Here's how the part is built. I have some questions about the finished solid (model axes, mm). Give positions to 0.01 mm unless a question says otherwise; leave off trailing zeros. Loops run counter-clockwise (first coordinate to the right, second up) from the corner with the lowest first, then second, coordinate; pieces in that order, holes last. Notation, with made-up numbers: (-27.5, -22.75) -> (-10.5, -22.75) arc R34 cw to (-10.5, 14.25) -> close; hole circle Ø5 at (54.5, -9). An arc over 180 degrees is marked (long way). Answer in a Markdown table with one row per item. Add a question column.
Item 1: We'd pull the mould along X, two halves only. Please class faces 1 (the face through (7.5, 1, 0)), 2 (the face through (-7.5, 1, 0)), 3 (the face through (-4.928, 0.811, -0.18)): released by +X, released by -X, zero draft, split by the parting line, or undercut.
Item 2: If we section it at A-A (z = 0): Write out the boundary of the cut face in (x, y).
Item 3: If we section it at B-B (x = -5.5): Write out the boundary of the cut face in (y, z), then the cut area to 3 significant figures.
Item 4: If I drill on line 1 (X direction, y = 0.9, z = 0); line 2 (Z direction, x = -5.5, y = 0.35); line 3 (Z direction, x = -5.25, y = 0.3), over which ranges is the centre line in solid material (lowest first)?
Item 5: If we section it at C-C (y = 0.4): Write out the boundary of the cut face in (x, z).
```python
from build123d import *

# Parameters (mm, degrees)
SKETCH1_W           = 15
SKETCH1_H           = 4
BOSS_EXTRUDE1_DEPTH = 1.6
SKETCH5_W           = 15
SKETCH5_H           = 1.6
BOSS_EXTRUDE4_DEPTH = 1.5
SKETCH6_W           = 15
SKETCH6_H           = 1.6
BOSS_EXTRUDE5_DEPTH = 0.9
SKETCH8_R           = 0.6
CUT_EXTRUDE1_DEPTH  = 10


with BuildPart() as part:
    # Sketch1 → Boss-Extrude1 (new body)
    with BuildSketch(Plane(origin=(0, 0, 0), x_dir=(1, 0, 0), z_dir=(0, 1, 0))):
        Rectangle(SKETCH1_W, SKETCH1_H)
    extrude(amount=BOSS_EXTRUDE1_DEPTH)

    # Sketch5 → Boss-Extrude4 (add)
    with BuildSketch(Plane.XY.offset(2)):
        with Locations((0, 0.8)):
            Rectangle(SKETCH5_W, SKETCH5_H)
    extrude(amount=BOSS_EXTRUDE4_DEPTH)

    # Sketch6 → Boss-Extrude5 (add)
    with BuildSketch(Plane(origin=(0, 0, -2), x_dir=(-1, 0, 0), z_dir=(0, 0, -1))):
        with Locations((0, 0.8)):
            Rectangle(SKETCH6_W, SKETCH6_H)
    extrude(amount=BOSS_EXTRUDE5_DEPTH)

    # Sketch8 → Cut-Extrude1 (cut)
    with BuildSketch(Plane(origin=(0, 1.6, 0), x_dir=(1, 0, 0), z_dir=(0, 1, 0))):
        with Locations((5.5, 0)):
            Circle(SKETCH8_R)
        with Locations((-5.5, 0)):
            Circle(SKETCH8_R)
    extrude(amount=-CUT_EXTRUDE1_DEPTH, mode=Mode.SUBTRACT)


solid = part.part
```
Recorded:
| question | item | result |
|---|---|---|
| 1 | face 1 | released by +X |
| 1 | face 2 | released by -X |
| 1 | face 3 | undercut |
| 2 | outline | (-7.5, 0) -> (-6.1, 0) -> (-6.1, 1.6) -> (-7.5, 1.6) -> close; (-4.9, 0) -> (4.9, 0) -> (4.9, 1.6) -> (-4.9, 1.6) -> close; (6.1, 0) -> (7.5, 0) -> (7.5, 1.6) -> (6.1, 1.6) -> close |
| 3 | outline | (0, -2.9) -> (1.6, -2.9) -> (1.6, -0.6) -> (0, -0.6) -> close; (0, 0.6) -> (1.6, 0.6) -> (1.6, 3.5) -> (0, 3.5) -> close |
| 3 | area | 8.32 mm^2 |
| 4 | line 1 | x = -7.5 to -6.1, -4.9 to 4.9, 6.1 to 7.5 |
| 4 | line 2 | z = -2.9 to -0.6, 0.6 to 3.5 |
| 4 | line 3 | z = -2.9 to -0.55, 0.55 to 3.5 |
| 5 | outline | (-7.5, -2.9) -> (7.5, -2.9) -> (7.5, 3.5) -> (-7.5, 3.5) -> close; hole circle Ø1.2 at (-5.5, 0); hole circle Ø1.2 at (5.5, 0) |
